```python
from build123d import *

# Parameters (mm, degrees)
BOSS_EXTRUDE1_DEPTH = 5
BOSS_EXTRUDE2_DEPTH = 2
SKETCH10_W          = 10
SKETCH10_H          = 5
BOSS_EXTRUDE7_DEPTH = 30
SKETCH11_R          = 3
BOSS_EXTRUDE8_DEPTH = 50
BOSS_EXTRUDE9_DEPTH = 5


with BuildPart() as part:
    # Sketch1 → Boss-Extrude1 (new body)
    with BuildSketch(Plane(origin=(0, 0, 0), x_dir=(1, 0, 0), z_dir=(0, 1, 0))):
        Polygon((-25, 15), (-25, -15), (-15, -15), (-13.266499161, -7), (13.266499161, -7), (15, -15), (25, -15), (25, 15), align=None)
    extrude(amount=BOSS_EXTRUDE1_DEPTH)

    # Sketch4 → Boss-Extrude2 (add)
    with BuildSketch(Plane.XZ):
        with BuildLine():
            Line((13.266499161, 7), (-13.266499161, 7))
            ThreePointArc((-13.266499161, 7), (-15, 0), (-13.266499161, -7))
            Line((-13.266499161, -7), (13.266499161, -7))
            ThreePointArc((13.266499161, -7), (14.560176637, -3.605725487), (15, 0))
            ThreePointArc((15, 0), (14.560176637, 3.605725487), (13.266499161, 7))
        make_face()
    extrude(amount=BOSS_EXTRUDE2_DEPTH)

    # Sketch10 → Boss-Extrude7 (add)
    with BuildSketch(Plane.XY.offset(15)):
        Polygon((-15, 10), (-15, 5), (-10, 10), align=None)
        with Locations((-20, 7.5)):
            Rectangle(SKETCH10_W, SKETCH10_H)
        Polygon((15, 10), (10, 10), (15, 5), align=None)
        with Locations((20, 7.5)):
            Rectangle(SKETCH10_W, SKETCH10_H)
    extrude(amount=-BOSS_EXTRUDE7_DEPTH)

    # Sketch11 → Boss-Extrude8 (add)
    with BuildSketch(Plane(origin=(25, 0, 0), x_dir=(0, 0, -1), z_dir=(1, 0, 0))):
        with BuildLine():
            Line((-7, -7), (-7, -2))
            Line((-7, -2), (7, -2))
            Line((7, -2), (7, -7))
            ThreePointArc((7, -7), (0, -14), (-7, -7))
        make_face()
        with Locations((0, -7)):
            Circle(SKETCH11_R, mode=Mode.SUBTRACT)
    extrude(amount=-BOSS_EXTRUDE8_DEPTH)

    # Sketch12 → Boss-Extrude9 (add)
    with BuildSketch(Plane(origin=(0, 0, -15), x_dir=(-1, 0, 0), z_dir=(0, 0, -1))):
        Polygon((-15, 5), (15, 5), (10, 10), (-10, 10), align=None)
    extrude(amount=-BOSS_EXTRUDE9_DEPTH)


solid = part.part
```
Model file for the job. Use its own axes, mm. A direction names the side the tool comes from. Round coordinates to 2 decimals unless told otherwise and drop trailing zeros. Loops run counter-clockwise (first coordinate to the right, second up) from the corner with the lowest first, then second, coordinate; pieces in that order, holes last. Notation, with made-up numbers: M 52.25,1 L 89.25,1 A20 cw 89.25,27 Z; hole C -18,32 d3. An arc over 180 degrees is marked long. Put each result on its own line as item: value. Start each with the question number.
Item 1: Cut at B-B (z = -8). List the corners of the cut face in (x, y), then the cut area to 3 significant figures.
Item 2: Drill centre lines: line 1 along Y through (x, z) = (-18.5, -0.75); line 2 along Y through (x, z) = (-8, 0); line 3 along Y through (x, z) = (21, -1). Where is each one in solid material? Low to high.
Item 3: Drop flat-ended pins along their axis: P1, Ø6, axis at x = 5.5, z = 3, coming from the +Y side; P2, Ø4, axis at x = -3, y = 7.5, coming from the +Z side; P3, Ø7.5, axis at x = -4.5, y = -4, coming from the -Z side. Give the stop position or say it passes through.
Item 4: Cut at A-A (x = 12). List the corners of the cut face in (y, z), then the cut area to 3 significant figures.
Item 5: Cut at D-D (x = -4). List the corners of the cut face in (y, z).
Item 6: Mould opens along Y. For faces 4 (the face through (0, -14, 0)), 5 (the face through (-14.145, 2.465, 11.056)), 6 (the face through (12, 8, 3)) say: released by +Y, released by -Y, zero draft, split by the parting line, or undercut.
Item 7: 3-axis set-ups, long thin cutter, end or side, ignore diameter. For faces 1 (the face through (0, -4, -7)), 2 (the face through (0, -2, 7)), 3 (the face through (0, 8, -10)): which of +Z, -Z, +X, -X, +Y, -Y reach the whole face in a straight line?
Item 8: Cut at C-C (y = 3.5). List the corners of the cut face in (x, z), then the cut area to 3 significant figures.
Answer block:
1. outline: M -25,0 L 25,0 L 25,10 L 10,10 L 15,5 L -15,5 L -10,10 L -25,10 Z
1. area: 375 mm2
2. line 1: -13.96 to -9.9, -4.1 to -2, 0 to 10
2. line 2: -14 to -10, -4 to 5
2. line 3: -13.93 to -9.83, -4.17 to -2, 0 to 10
3. P1: y = 5
3. P2: z = -10
3. P3: z = -7
4. outline: M -7,-7 L 0,-7 L 0,-15 L 10,-15 L 10,15 L 8,15 L 8,-10 L 5,-10 L 5,7 L -7,7 A7 ccw Z; hole C -7,0 d6
4. area: 332 mm2
5. outline: M -7,-7 L 0,-7 L 0,-15 L 10,-15 L 10,-10 L 5,-10 L 5,7 L -7,7 A7 ccw Z; hole C -7,0 d6
6. face 4: released by -Y
6. face 5: zero draft
6. face 6: undercut
7. face 1: -Z, +X, -X, -Y
7. face 2: +Z, -Y
7. face 3: +Z
8. outline: M -25,-15 L 25,-15 L 25,15 L 15,15 L 13.27,7 L -13.27,7 L -15,15 L -25,15 Z
8. area: 1,270 mm2
